from build123d import *

# Parameters (mm, degrees)
BOSS_EXTRUDE1_DEPTH                            = 4
CBORE_FOR_4_SOCKET_HEAD_CAP_SCREW1_D           = 3.2639
CBORE_FOR_4_SOCKET_HEAD_CAP_SCREW1_DEPTH       = 9.019425513
CBORE_FOR_4_SOCKET_HEAD_CAP_SCREW1_CBORE_D     = 5.55752
CBORE_FOR_4_SOCKET_HEAD_CAP_SCREW1_CBORE_DEPTH = 2.8448
CBORE_FOR_4_SOCKET_HEAD_CAP_SCREW1_TIP         = 0.980574487
CBORE_FOR_8_SOCKET_HEAD_CAP_SCREW1_D           = 4.4958
CBORE_FOR_8_SOCKET_HEAD_CAP_SCREW1_DEPTH       = 8.649325414
CBORE_FOR_8_SOCKET_HEAD_CAP_SCREW1_CBORE_D     = 7.9375
CBORE_FOR_8_SOCKET_HEAD_CAP_SCREW1_CBORE_DEPTH = 4.1656
CBORE_FOR_8_SOCKET_HEAD_CAP_SCREW1_TIP         = 1.350674586


with BuildPart() as part:
    # Sketch1 → Boss-Extrude1 (new body, symmetric)
    with BuildSketch(Plane.XY):
        with BuildLine():
            ThreePointArc((-44.12938743, -0.647051637), (-43.384473284, -9.954325443), (-34.443470177, -7.263841056))
            ThreePointArc((-34.443470177, -7.263841056), (-30.155368055, -2.36099743), (-23.757529046, -1.138969828))
            ThreePointArc((-23.757529046, -1.138969828), (-22.961581659, -1.18930409), (-22.167756654, -1.112442901))
            ThreePointArc((-22.167756654, -1.112442901), (-12.010862121, -1.048885846), (-2.414899511, -4.378157187))
            ThreePointArc((-2.414899511, -4.378157187), (0, -5), (2.414899511, -4.378157187))
            ThreePointArc((2.414899511, -4.378157187), (12.010862121, -1.048885846), (22.167756654, -1.112442901))
            ThreePointArc((22.167756654, -1.112442901), (22.961581659, -1.18930409), (23.757529046, -1.138969828))
            ThreePointArc((23.757529046, -1.138969828), (30.155368055, -2.36099743), (34.443470177, -7.263841056))
            ThreePointArc((34.443470177, -7.263841056), (43.384473284, -9.954325443), (44.12938743, -0.647051637))
            ThreePointArc((44.12938743, -0.647051637), (34.621269329, 5.779365543), (23.545617652, 8.78487507))
            ThreePointArc((23.545617652, 8.78487507), (22.042434881, 8.708455183), (20.630100489, 8.188157187))
            ThreePointArc((20.630100489, 8.188157187), (11.034137879, 4.858885846), (0.877243346, 4.922442901))
            ThreePointArc((0.877243346, 4.922442901), (0, 5), (-0.877243346, 4.922442901))
            ThreePointArc((-0.877243346, 4.922442901), (-11.034137879, 4.858885846), (-20.630100489, 8.188157187))
            ThreePointArc((-20.630100489, 8.188157187), (-22.042434881, 8.708455183), (-23.545617652, 8.78487507))
            ThreePointArc((-23.545617652, 8.78487507), (-34.621269329, 5.779365543), (-44.12938743, -0.647051637))
        make_face()
    extrude(amount=BOSS_EXTRUDE1_DEPTH, both=True)

    # CBORE for #4 Socket Head Cap Screw1
    with Locations(Plane.XY.offset(4)):
        with Locations((-23.045, 3.81), (0, 0), (23.045, 3.81)):
            CounterBoreHole(CBORE_FOR_4_SOCKET_HEAD_CAP_SCREW1_D / 2, CBORE_FOR_4_SOCKET_HEAD_CAP_SCREW1_CBORE_D / 2, CBORE_FOR_4_SOCKET_HEAD_CAP_SCREW1_CBORE_DEPTH, depth=CBORE_FOR_4_SOCKET_HEAD_CAP_SCREW1_DEPTH)
            with Locations((0, 0, -(CBORE_FOR_4_SOCKET_HEAD_CAP_SCREW1_DEPTH + CBORE_FOR_4_SOCKET_HEAD_CAP_SCREW1_TIP / 2))):  # 118° drill point
                Cone(0, CBORE_FOR_4_SOCKET_HEAD_CAP_SCREW1_D / 2, CBORE_FOR_4_SOCKET_HEAD_CAP_SCREW1_TIP, mode=Mode.SUBTRACT)

    # CBORE for #8 Socket Head Cap Screw1
    with Locations(Plane(origin=(0, 0, -4), x_dir=(-1, 0, 0), z_dir=(0, 0, -1))):
        with Locations((-40, -5), (40, -5)):
            CounterBoreHole(CBORE_FOR_8_SOCKET_HEAD_CAP_SCREW1_D / 2, CBORE_FOR_8_SOCKET_HEAD_CAP_SCREW1_CBORE_D / 2, CBORE_FOR_8_SOCKET_HEAD_CAP_SCREW1_CBORE_DEPTH, depth=CBORE_FOR_8_SOCKET_HEAD_CAP_SCREW1_DEPTH)
            with Locations((0, 0, -(CBORE_FOR_8_SOCKET_HEAD_CAP_SCREW1_DEPTH + CBORE_FOR_8_SOCKET_HEAD_CAP_SCREW1_TIP / 2))):  # 118° drill point
                Cone(0, CBORE_FOR_8_SOCKET_HEAD_CAP_SCREW1_D / 2, CBORE_FOR_8_SOCKET_HEAD_CAP_SCREW1_TIP, mode=Mode.SUBTRACT)


solid = part.part
The model under review builds one solid part; all positions refer to its coordinate system, in mm. A direction names the side the tool comes from. Give positions to 0.01 mm unless a question says otherwise; leave off trailing zeros. Write each loop counter-clockwise with the first axis right and the second up, starting at its lowest first coordinate (ties: lowest second). Pieces come first, ordered by that corner, then holes.
1. Tool access review of faces 1 (the flat face through (0, -2, 1.155)), 2 (the cylindrical face through (34.77, 5.71, 0.06)): name each direction out of +Z, -Z, +X, -X, +Y, -Y from which nothing blocks a thin tool from reaching the whole face with its end or side.
2. Add section C-C, the plane x = 0. Write out the cut boundary in (y, z).
3. Wall thickness on L1, parallel to X at y = -5.25, z = 2.25; L2, parallel to X at y = -9.5, z = 2.5; L3, parallel to X at y = 2, z = 1.5: over which ranges is each line inside the solid? List them lowest first.
4. Add section D-D, the plane x = -29. Write out the cut boundary in (y, z), plus the area to 3 significant figures.
5. Add section A-A, the plane x = 40. Write out the cut boundary in (y, z).
6. Add section B-B, the plane z = -1.75. Write out the cut boundary in (x, y) (1 decimal), plus the area to 3 significant figures.
7. Draft analysis for pull direction Y (two halves, no side actions). For faces 3 (the flat face through (0, 3, -4)), 4 (the cylindrical face through (30.075, -2.315, 0.056)), 5 (the cylindrical face through (-0.602, -2.713, 2.598)), state which applies: +Y half, -Y half, draft (parallel to the pull), parting line (faces both ways), or undercut.
8. For P1, Ø4, axis at x = 34, z = 0, coming from the +Y side; P2, Ø4, axis at x = -40.5, y = -6, coming from the -Z side; P3, Ø2, axis at y = -2, z = 0, coming from the +X side, all flat-tipped, find the tip position at first contact; note any pin that passes through.
Worked answers:
1. face 1: +Z
1. face 2: +Z, -Z, +X, +Y
2. outline: (-5, -4) - (-1.63, -4) - (-1.63, 1.16) - (-2.78, 1.16) - (-2.78, 4) - (-5, 4) - close; (1.63, -4) - (5, -4) - (5, 4) - (2.78, 4) - (2.78, 1.16) - (1.63, 1.16) - close
3. L1: x = -45.99 to -42.23, -37.77 to -33.34, 33.34 to 37.77, 42.23 to 45.99
3. L2: x = -43.97 to -36.03, 36.03 to 43.97
3. L3: x = -40.99 to -25.15, -20.94 to -1.93, 1.93 to 20.94, 25.15 to 40.99
4. outline: (-1.79, -4) - (7.79, -4) - (7.79, 4) - (-1.79, 4) - close
4. area: 76.7 mm2
5. outline: (-11, -4) - (-8.97, -4) - (-8.97, 0.17) - (-7.25, 0.17) - (-7.25, 4) - (-11, 4) - close; (-2.75, 0.17) - (-1.03, 0.17) - (-1.03, -4) - (2.71, -4) - (2.71, 4) - (-2.75, 4) - close
6. outline: (-44.1, -0.6) arc R6 ccw (long way) to (-34.4, -7.3) arc R10 cw to (-23.8, -1.1) arc R5 ccw to (-22.2, -1.1) arc R30 cw to (-2.4, -4.4) arc R5 ccw to (2.4, -4.4) arc R30 cw to (22.2, -1.1) arc R5 ccw to (23.8, -1.1) arc R10 cw to (34.4, -7.3) arc R6 ccw (long way) to (44.1, -0.6) arc R35 ccw to (23.5, 8.8) arc R5 ccw to (20.6, 8.2) arc R30 cw to (0.9, 4.9) arc R5 ccw to (-0.9, 4.9) arc R30 cw to (-20.6, 8.2) arc R5 ccw to (-23.5, 8.8) arc R35 ccw to start; hole circle Ø7.9 at (-40, -5); hole circle Ø3.3 at (-23, 3.8); hole circle Ø3.3 at (0, 0); hole circle Ø3.3 at (23, 3.8); hole circle Ø7.9 at (40, -5)
6. area: 736 mm2
7. face 3: draft
7. face 4: -Y half
7. face 5: undercut
8. P1: stops at y = 6.85
8. P2: stops at z = 0.17
8. P3: stops at x = 45.66
